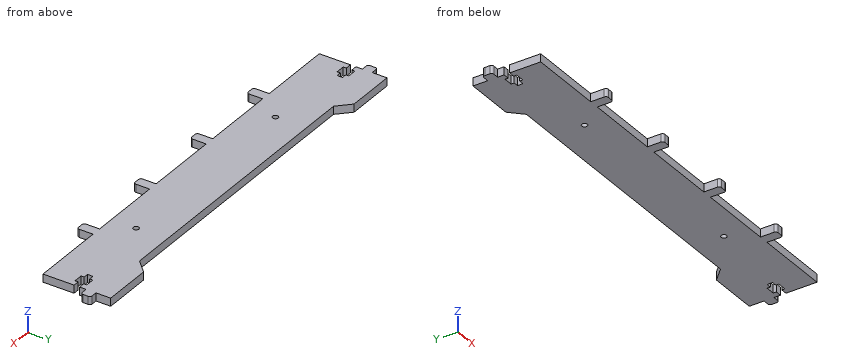
Autodesk Inventor part; units mm, degrees
ref_plane "YZ Plane" through (0, 0, 0) normal (1, 0, 0) x (0, 1, 0)
ref_plane "XZ Plane" through (0, 0, 0) normal (0, 1, 0) x (-1, 0, 0)
ref_plane "XY Plane" through (0, 0, 0) normal (0, 0, 1) x (1, 0, 0)
sketch "Sketch1" plane through (0, 0, 0) normal (0, 0, 1) x (1, 0, 0)
  line L0 (0, 0) -> (336, 0)
  line L1 (336, 0) -> (336, 55)
  line L2 (0, 55) -> (0, 0)
  line L3 (40, 55) -> (50, 45)
  line L4 (50, 45) -> (286, 45)
  line L5 (286, 45) -> (296, 55)
  line L6 (336, 55) -> (296, 55)
  line L7 (40, 55) -> (0, 55)
  dimension "d0" = 336
  dimension "d1" = 55
  dimension "d2" = 45
  dimension "d3" = 40
  dimension "d4" = 10
  dimension "d5" = 40
extrude "Extrusion1" add sketch "Sketch1" along normal blind 6.5
sketch "Sketch2" plane through (0, 0, 6.5) normal (0, 0, 1) x (1, 0, 0)
  line L0 (0, 0) -> (336, 0)
  line L1 (286, 45) -> (50, 45)
  line L2 (0, 55) -> (0, 0)
  line L3 (0, 25.25) -> (0, 29.75)
  line L4 (16.3, 29.75) -> (16.3, 25.25)
  line L5 (5, 32.25) -> (12.3, 32.25)
  line L6 (12.3, 22.75) -> (5, 22.75)
  line L7 (0, 29.75) -> (5, 29.75)
  line L8 (12.3, 29.75) -> (16.3, 29.75)
  line L9 (16.3, 25.25) -> (12.3, 25.25)
  line L10 (5, 25.25) -> (0, 25.25)
  line L11 (5, 22.75) -> (5, 25.25)
  line L12 (5, 29.75) -> (5, 32.25)
  line L13 (12.3, 32.25) -> (12.3, 29.75)
  line L14 (12.3, 25.25) -> (12.3, 22.75)
  line L15 (168, 0) -> (168, 45) construction
  line L16 (336, 25.25) -> (336, 29.75)
  line L17 (319.7, 29.75) -> (319.7, 25.25)
  line L18 (331, 32.25) -> (323.7, 32.25)
  line L19 (323.7, 22.75) -> (331, 22.75)
  line L20 (336, 29.75) -> (331, 29.75)
  line L21 (323.7, 29.75) -> (319.7, 29.75)
  line L22 (319.7, 25.25) -> (323.7, 25.25)
  line L23 (331, 25.25) -> (336, 25.25)
  line L24 (331, 22.75) -> (331, 25.25)
  line L25 (331, 29.75) -> (331, 32.25)
  line L26 (323.7, 32.25) -> (323.7, 29.75)
  line L27 (323.7, 25.25) -> (323.7, 22.75)
  point P0 (0, 27.5)
  point P1 (0, 27.5)
  point P2 (336, 27.5)
  point P3 (336, 27.5)
  dimension "d8" = 4.5
  dimension "d9" = 2.5
  dimension "d10" = 2.5
  dimension "d11" = 5
  dimension "d12" = 7.3
  dimension "d13" = 4
extrude "Extrusion2" cut sketch "Sketch2" against normal through all
sketch "Sketch3" plane through (0, 0, 6.5) normal (0, 0, 1) x (1, 0, 0)
  line L0 (0, 25.25) -> (0, 0)
  line L1 (0, 0) -> (336, 0)
  line L2 (336, 0) -> (336, 25.25)
  line L3 (336, 29.75) -> (336, 55)
  line L4 (0, 55) -> (0, 29.75)
  line L5 (16.3, 29.75) -> (16.3, 25.25)
  line L6 (0, 43) -> (-4.5, 43)
  line L7 (-6.5, 41) -> (-6.5, 37)
  line L8 (-4.5, 35) -> (0, 35)
  line L9 (0, 35) -> (0, 43)
  line L10 (0, 20) -> (-4.5, 20)
  line L11 (-6.5, 18) -> (-6.5, 14)
  line L12 (-4.5, 12) -> (0, 12)
  line L13 (0, 12) -> (0, 20)
  arc A0 (-4.5, 43) -> (-6.5, 41) centre (-4.5, 41) ccw
  arc A1 (-6.5, 37) -> (-4.5, 35) centre (-4.5, 37) ccw
  arc A2 (-4.5, 20) -> (-6.5, 18) centre (-4.5, 18) ccw
  arc A3 (-6.5, 14) -> (-4.5, 12) centre (-4.5, 14) ccw
  line L14 (336, 43) -> (340.5, 43)
  line L15 (342.5, 41) -> (342.5, 37)
  line L16 (340.5, 35) -> (336, 35)
  line L17 (336, 35) -> (336, 43)
  line L18 (336, 20) -> (340.5, 20)
  line L19 (342.5, 18) -> (342.5, 14)
  line L20 (340.5, 12) -> (336, 12)
  line L21 (336, 12) -> (336, 20)
  arc A4 (342.5, 41) -> (340.5, 43) centre (340.5, 41) ccw
  arc A5 (340.5, 35) -> (342.5, 37) centre (340.5, 37) ccw
  arc A6 (342.5, 18) -> (340.5, 20) centre (340.5, 18) ccw
  arc A7 (340.5, 12) -> (342.5, 14) centre (340.5, 14) ccw
  line L22 (198.4, 0) -> (206.4, 0)
  line L23 (206.4, 0) -> (206.4, -11)
  line L24 (204.4, -13) -> (200.4, -13)
  line L25 (198.4, -11) -> (198.4, 0)
  line L26 (137.6, 0) -> (129.6, 0)
  line L27 (129.6, 0) -> (129.6, -11)
  line L28 (131.6, -13) -> (135.6, -13)
  line L29 (137.6, -11) -> (137.6, 0)
  line L30 (60.8, 0) -> (68.8, 0)
  line L31 (68.8, 0) -> (68.8, -11)
  line L32 (66.8, -13) -> (62.8, -13)
  line L33 (60.8, -11) -> (60.8, 0)
  line L34 (267.2, 0) -> (275.2, 0)
  line L35 (275.2, 0) -> (275.2, -11)
  line L36 (273.2, -13) -> (269.2, -13)
  line L37 (267.2, -11) -> (267.2, 0)
  arc A8 (60.8, -11) -> (62.8, -13) centre (62.8, -11) ccw
  arc A9 (66.8, -13) -> (68.8, -11) centre (66.8, -11) ccw
  arc A10 (129.6, -11) -> (131.6, -13) centre (131.6, -11) ccw
  arc A11 (135.6, -13) -> (137.6, -11) centre (135.6, -11) ccw
  arc A12 (198.4, -11) -> (200.4, -13) centre (200.4, -11) ccw
  arc A13 (204.4, -13) -> (206.4, -11) centre (204.4, -11) ccw
  arc A14 (267.2, -11) -> (269.2, -13) centre (269.2, -11) ccw
  arc A15 (273.2, -13) -> (275.2, -11) centre (273.2, -11) ccw
  line L38 (68.8, -5.5) -> (129.6, -5.5) construction
  line L39 (137.6, -5.5) -> (198.4, -5.5) construction
  line L40 (206.4, -5.5) -> (267.2, -5.5) construction
  line L41 (275.2, -5.5) -> (336, -5.5) construction
  line L42 (60.8, -5.5) -> (0, -5.5) construction
  point P0 (16.3, 27.5)
  point P1 (168, 0)
  dimension "d16" = 2
  dimension "d17" = 8
  dimension "d18" = 8
  dimension "d19" = 15
  dimension "d20" = 7.5
  dimension "d21" = 6.5
  dimension "d22" = 2
  dimension "d23" = 6.5
  dimension "d24" = 2
  dimension "d25" = 8
  dimension "d26" = 8
  dimension "d27" = 8
  dimension "d28" = 8
  dimension "d29" = 13
extrude "Extrusion3" add sketch "Sketch3" against normal blind 6.5
sketch "Sketch4" plane through (0, 0, 6.5) normal (0, 0, 1) x (1, 0, 0)
  line L0 (0, 20) -> (-4.5, 20)
  arc A0 (-4.5, 20) -> (-6.5, 18) centre (-4.5, 18) ccw
  line L1 (-6.5, 18) -> (-6.5, 14)
  arc A1 (-6.5, 14) -> (-4.5, 12) centre (-4.5, 14) ccw
  line L2 (-4.5, 12) -> (0, 12)
  line L3 (336, 12) -> (340.5, 12)
  arc A2 (340.5, 12) -> (342.5, 14) centre (340.5, 14) ccw
  line L4 (342.5, 14) -> (342.5, 18)
  arc A3 (342.5, 18) -> (340.5, 20) centre (340.5, 18) ccw
  line L5 (340.5, 20) -> (336, 20)
  line L6 (5, 22.75) -> (5, 25.25)
  line L7 (0, 20) -> (0, 12)
  line L8 (336, 20) -> (336, 12)
extrude "Extrusion4" cut sketch "Sketch4" against normal through all
sketch "Sketch5" plane through (0, 0, 6.5) normal (0, 0, 1) x (1, 0, 0)
  line L0 (0, 25.25) -> (0, 0)
  line L1 (0, 0) -> (60.8, 0)
  line L2 (336, 0) -> (336, 25.25)
  circle A0 centre (83.25, 20) radius 2.25
  circle A1 centre (252.75, 20) radius 2.25
  dimension "d34" = 4.5
  dimension "d35" = 20
  dimension "d36" = 83.25
  dimension "d37" = 83.25
extrude "Extrusion5" cut sketch "Sketch5" against normal through all
equation "\"d5\" = d3"
equation "\"d23\" = d21"
equation "\"d37\" = d36"
properties part number "frame_brace_top" material "Plywood, Finish"
Could you check a few things on this model? Use its own coordinates, in mm. Round coordinates to 2 decimals unless told otherwise and drop trailing zeros. Loops run counter-clockwise (first coordinate to the right, second up) from the corner with the lowest first, then second, coordinate; pieces in that order, holes last. Notation, with made-up numbers: M 55.25,39.5 L 106.25,39.5 A20 ccw 106.25,51.5 Z; hole C 17,-35.75 d7. An arc over 180 degrees is marked long. Answer as CSV lines item,"result".
1) For pin 1 Ø1.5 at (x, y) = (30.5, 17.5) entering from -Z; pin 2 Ø3 at (y, z) = (45, 0.5) entering from +X; pin 3 Ø1.5 at (x, z) = (168, 5.5) entering from +Y; pin 4 Ø2.5 at (x, y) = (83.25, 20) entering from -Z, each with a flat end and sliding along its axis, tell me the tip position at first contact or that it passes through.
From the geometry:
pin 1,"z = 0"
pin 2,"x = 336"
pin 3,"y = 45"
pin 4,"through"
2) Imagine slicing it at B-B on x = 177. List the corners of the cut face in (y, z) for me, and give its area (4 significant figures).
From the geometry:
outline,"M 0,0 L 45,0 L 45,6.5 L 0,6.5 Z"
area,"292.5 mm^2"
3) If I drill on probe 1 along X at (y, z) = (-5, 2); probe 2 along Y at (x, z) = (83.25, 5.25); probe 3 along Y at (x, z) = (190.5, 1.5), over which ranges is the centre line in solid material (lowest first)?
From the geometry:
probe 1,"60.8 to 68.8, 129.6 to 137.6, 198.4 to 206.4, 267.2 to 275.2"
probe 2,"0 to 17.75, 22.25 to 45"
probe 3,"0 to 45"
4) Imagine slicing it at A-A on z = 2.25. Count the separate pieces of the cut face and the enclosed holes in it, and give its area (3 significant figures).
From the geometry:
separate pieces,"1"
enclosed holes,"2"
area,"16,300 mm^2"
